Source: CAD feature listing. Evaluate the final solid. Frame: model axes, mm. Face numbers are marked on the shaded views. A direction names the side the tool comes from. Give positions to 0.01 mm unless a question says otherwise; leave off trailing zeros. Order: outer loops, then holes, each group sorted by start corner. A loop starts at its lowest first (then second) coordinate and runs counter-clockwise, first axis right, second up. Notation, with made-up numbers: (16.25, -35) - (64.25, -35) arc R13 ccw to (64.25, -22) - close; hole circle Ø10 at (-32, -24.5). An arc over 180 degrees is marked (long way). Use CSV: the item, a comma, the result in double quotes.
Autodesk Inventor part; units mm, degrees
ref_plane "YZ Plane" through (0, 0, 0) normal (1, 0, 0) x (0, 1, 0)
ref_plane "XZ Plane" through (0, 0, 0) normal (0, 1, 0) x (-1, 0, 0)
ref_plane "XY Plane" through (0, 0, 0) normal (0, 0, 1) x (1, 0, 0)
sketch "Sketch1" plane through (0, 0, 0) normal (0, 1, 0) x (-1, 0, 0)
  circle A0 centre (0, 0) radius 5
  dimension "d0" = 10
extrude "Extrusion1" add sketch "Sketch1" along normal blind 4
sketch "Sketch2" plane through (0, 4, 0) normal (0, 1, 0) x (1, 0, 0)
  circle A0 centre (0, 0) radius 3.1115
  dimension "d3" = 6.223
extrude "Extrusion2" add sketch "Sketch2" along normal blind 19.5
sketch "Sketch3" plane through (0, 23.5, 0) normal (0, 1, 0) x (1, 0, 0)
  circle A0 centre (0, 0) radius 1.4
  dimension "d6" = 2.8
extrude "Extrusion3" cut sketch "Sketch3" against normal through all
properties part number "BoltandHole12"
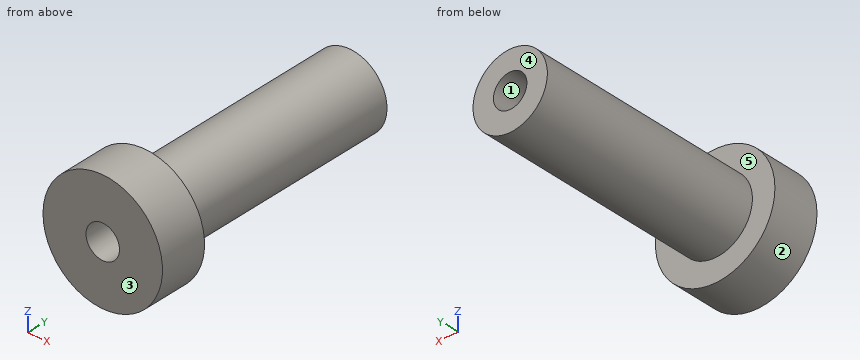
Item 1: Mould query, pull axis Z, two halves, no side actions, for the marked faces 1, 2 and 3. Classes: released by +Z, released by -Z, zero draft, split by the parting line, or undercut.
Filled in:
face 1,"undercut"
face 2,"split by the parting line"
face 3,"zero draft"
Item 2: Section C-C on y = 6.5. Return the cut outline in (x, z), then the cut area to 3 significant figures.
Filled in:
outline,"circle Ø6.22 at (0, 0); hole circle Ø2.8 at (0, 0)"
area,"24.3 mm2"
Item 3: Section B-B on x = 0. Return the cut outline in (y, z), then the cut area to 3 significant figures.
Filled in:
outline,"(0, -5) - (4, -5) - (4, -3.11) - (23.5, -3.11) - (23.5, -1.4) - (0, -1.4) - close; (0, 1.4) - (23.5, 1.4) - (23.5, 3.11) - (4, 3.11) - (4, 5) - (0, 5) - close"
area,"95.5 mm2"
Item 4: First-contact query: pin 1 (3 mm diameter, centred on y = 3, z = 4, fed in from -X); pin 2 (2 mm diameter, centred on x = 0, y = 7, fed in from -Z); pin 3 (2 mm diameter, centred on x = 1.5, y = 17, fed in from +Z). Flat tips, straight axial feed; report the tip coordinate or a pass-through.
Filled in:
pin 1,"stops at x = -4.33"
pin 2,"stops at z = -3.11"
pin 3,"stops at z = 3.07"
Item 5: Material intervals for line 1 (X direction, y = 12.75, z = 0); line 2 (Y direction, x = -2, z = 4.25), sorted ascending. Write a range as from..to.
Filled in:
line 1,"x = -3.11..-1.4, 1.4..3.11"
line 2,"y = 0..4"
Item 6: Section A-A on z = 0. Return the cut outline in (x, y), then the cut area to 3 significant figures.
Filled in:
outline,"(-5, 0) - (-1.4, 0) - (-1.4, 23.5) - (-3.11, 23.5) - (-3.11, 4) - (-5, 4) - close; (1.4, 0) - (5, 0) - (5, 4) - (3.11, 4) - (3.11, 23.5) - (1.4, 23.5) - close"
area,"95.5 mm2"
Item 7: Set-up query: the marked faces 4 and 5. Return all of +Z, -Z, +X, -X, +Y, -Y with unobstructed straight access to the full face (end or side cutting, diameter ignored); none if empty.
Filled in:
face 4,"+Z, -Z, +X, -X, +Y"
face 5,"+Y"
Item 8: Section D-D on z = 2. Return the cut outline in (x, y).
Filled in:
outline,"(-4.58, 0) - (4.58, 0) - (4.58, 4) - (2.38, 4) - (2.38, 23.5) - (-2.38, 23.5) - (-2.38, 4) - (-4.58, 4) - close"
